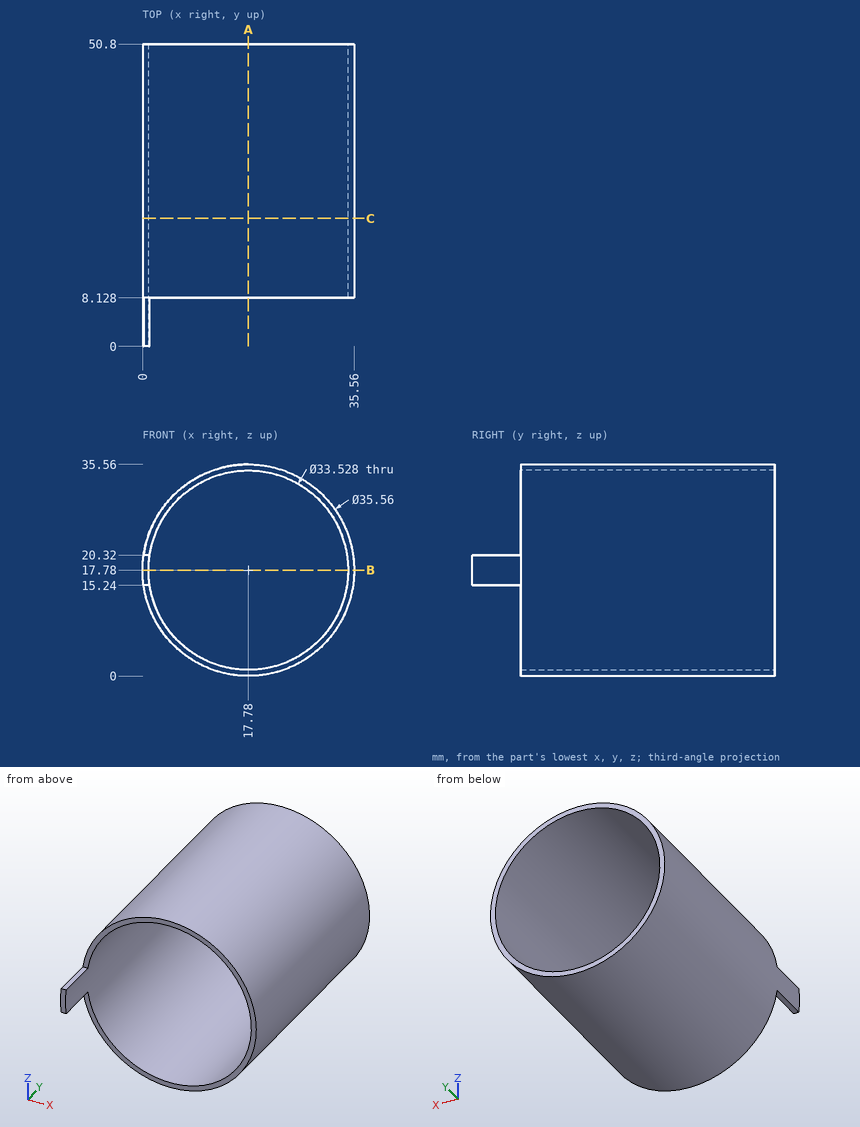
The drawing under review shows one solid part. Ordinate dimensions are in mm from its lowest x, y, z. Round coordinates to 2 decimals unless told otherwise and drop trailing zeros. Order: outer loops, then holes, each group sorted by start corner. A loop starts at its lowest first (then second) coordinate and runs counter-clockwise, first axis right, second up. Notation, with made-up numbers: (18.25, 25) -> (36.25, 25) arc R27 ccw to (36.25, 57) -> close; hole circle Ø3 at (83, -7.5). An arc over 180 degrees is marked (long way). Return JSON: item names as keys, results as strings.
1. Insertion check: P1, Ø0.5, axis at x = 0.5, y = 2.5, coming from the +Z side; P2, Ø4, axis at x = 26.5, y = 36.5, coming from the -Z side; P3, Ø6, axis at y = 11.5, z = 4.5, coming from the -X side. Each pin has a flat end and moves straight along its axis. Give the tip position at first contact, or say it passes through.
Answer block:
{"P1": "stops at z = 20.32", "P2": "stops at z = 1.32", "P3": "stops at x = 3.27"}
2. Take a section at C-C (y = 21.5). Write out the cut boundary in (x, z), then the cut area to 3 significant figures.
Answer block:
{"outline": "circle Ø35.56 at (17.78, 17.78); hole circle Ø33.53 at (17.78, 17.78)", "area": "110 mm²"}
3. Take a section at B-B (z = 17.78). Write out the cut boundary in (x, y).
Answer block:
{"outline": "(0, 0) -> (1.02, 0) -> (1.02, 50.8) -> (0, 50.8) -> close; (34.54, 8.13) -> (35.56, 8.13) -> (35.56, 50.8) -> (34.54, 50.8) -> close"}
4. For L1, parallel to Z at x = 17.78, y = 15.5; L2, parallel to Z at x = 27, y = 15, list the stretches that pass through material, from the lowest coordinate up. Write a range as [from, to].
Answer block:
{"L1": "z = [0, 1.02], [34.54, 35.56]", "L2": "z = [2.58, 3.78], [31.78, 32.98]"}
5. Take a section at A-A (x = 17.78). Write out the cut boundary in (y, z), then the cut area to 3 significant figures.
Answer block:
{"outline": "(8.13, 0) -> (50.8, 0) -> (50.8, 1.02) -> (8.13, 1.02) -> close; (8.13, 34.54) -> (50.8, 34.54) -> (50.8, 35.56) -> (8.13, 35.56) -> close", "area": "86.7 mm²"}
